from build123d import *

# Parameters (mm, degrees)
SKETCH1_R           = 2.5
SKETCH1_R_2         = 10.5
SKETCH1_R_3         = 1.5
BOSS_EXTRUDE1_DEPTH = 4


with BuildPart() as part:
    # Sketch1 → Boss-Extrude1 (new body)
    with BuildSketch(Plane(origin=(0, 0, 0), x_dir=(1, 0, 0), z_dir=(0, 1, 0))):
        with BuildLine():
            Line((-27, -75), (27, -75))
            ThreePointArc((27, -75), (43.263455967, -68.263455967), (50, -52))
            Line((50, -52), (50, 52))
            ThreePointArc((50, 52), (43.263455967, 68.263455967), (27, 75))
            Line((27, 75), (-27, 75))
            ThreePointArc((-27, 75), (-43.263455967, 68.263455967), (-50, 52))
            Line((-50, 52), (-50, -52))
            ThreePointArc((-50, -52), (-43.263455967, -68.263455967), (-27, -75))
        make_face()
        with Locations((-36, 61)):
            Circle(SKETCH1_R, mode=Mode.SUBTRACT)
        with Locations((-36, -61)):
            Circle(SKETCH1_R, mode=Mode.SUBTRACT)
        with Locations((36, -61)):
            Circle(SKETCH1_R, mode=Mode.SUBTRACT)
        with Locations((36, 61)):
            Circle(SKETCH1_R, mode=Mode.SUBTRACT)
        with Locations((0, 38)):
            Circle(SKETCH1_R, mode=Mode.SUBTRACT)
        with Locations((0, 15.5)):
            Circle(SKETCH1_R_2, mode=Mode.SUBTRACT)
        with Locations((15.5, 31)):
            Circle(SKETCH1_R_3, mode=Mode.SUBTRACT)
        with Locations((-15.5, 31)):
            Circle(SKETCH1_R_3, mode=Mode.SUBTRACT)
        with Locations((-15.5, 0)):
            Circle(SKETCH1_R_3, mode=Mode.SUBTRACT)
        with Locations((15.5, 0)):
            Circle(SKETCH1_R_3, mode=Mode.SUBTRACT)
    extrude(amount=BOSS_EXTRUDE1_DEPTH)


solid = part.part
Design review of the part built by this model. Coordinates are the model's own, in mm. Round coordinates to 2 decimals unless told otherwise and drop trailing zeros. Write each loop counter-clockwise with the first axis right and the second up, starting at its lowest first coordinate (ties: lowest second). Pieces come first, ordered by that corner, then holes. Notation, with made-up numbers: (-27, -24.75) -> (-10, -24.75) arc R15 ccw to (-10, -10.75) -> close; hole circle Ø4 at (33, 41). An arc over 180 degrees is marked (long way). One line per item, written item: value. Start each with the question number.
Q1. Add section C-C (z = -15.5). Give the boundary of the cut face in (x, y).
Q2. Add section A-A (x = 15.5). Give the boundary of the cut face in (y, z).
Q3. Insertion check: P1, Ø1, axis at y = 1, z = -56.5, coming from the +X side. The pin has a flat end and moves straight along its axis. Give the tip position at first contact, or say it passes through.
Q4. Add section D-D (y = 1.85). State how many separate pieces and enclosed holes the cut face has, then the cut area to 3 significant figures.
Q5. To check wall thickness, follow probe 1 along Z at (x, y) = (0, 2.25); probe 2 along X at (y, z) = (2.15, 0); probe 3 along X at (y, z) = (1.1, -38). State the ranges of each line that lie inside material, in increasing order.
Q6. Add section B-B (z = -31). Give the boundary of the cut face in (x, y), then the cut area to 3 significant figures.
Q7. The part is to be moulded in two halves that separate along Z. For faces 1 (the face through (0, 2, -75)), 2 (the face through (-33.69, 1.97, -60.04)), 3 (the face through (14, 2, 0)), 4 (the face through (-50, 2, -1)), say which applies: pulls with the +Z half, pulls with the -Z half, needs draft (parallel to the pull), parting line crosses it, or undercut.
Response:
1. outline: (-50, 0) -> (-10.5, 0) -> (-10.5, 4) -> (-50, 4) -> close; (10.5, 0) -> (50, 0) -> (50, 4) -> (10.5, 4) -> close
2. outline: (0, -75) -> (4, -75) -> (4, -32.5) -> (0, -32.5) -> close; (0, -29.5) -> (4, -29.5) -> (4, -1.5) -> (0, -1.5) -> close; (0, 1.5) -> (4, 1.5) -> (4, 75) -> (0, 75) -> close
3. P1: stops at x = 49.65
4. separate pieces: 1
4. enclosed holes: 10
4. area: 14,100 mm^2
5. probe 1: z = -75 to -40.5, -35.5 to -26, -5 to 75
5. probe 2: x = -50 to -17, -14 to 14, 17 to 50
5. probe 3: x = -50 to -2.5, 2.5 to 50
6. outline: (-50, 0) -> (-17, 0) -> (-17, 4) -> (-50, 4) -> close; (-14, 0) -> (14, 0) -> (14, 4) -> (-14, 4) -> close; (17, 0) -> (50, 0) -> (50, 4) -> (17, 4) -> close
6. area: 376 mm^2
7. face 1: pulls with the -Z half
7. face 2: undercut
7. face 3: undercut
7. face 4: needs draft
